from build123d import *

# Parameters (mm, degrees)
F0_W         = 119.1
F0_H         = 80
F1_DEPTH     = 5
F3_DEPTH     = 63.1
F4_W         = 6.8
F4_H         = 2
F4_W_2       = 7
F4_W_3       = 6.5
F5_DEPTH     = 4
F6_W         = 47.8
F6_H         = 2
F7_DEPTH     = 4
F8_W         = 0.5
F8_H         = 68
F9_DEPTH     = 25
F10_W        = 80
F10_H        = 5
F11_DEPTH    = 2
F12_W        = 2
F12_H        = 32.5577612221
F12_H_2      = 47.4422387779
F13_DEPTH    = 4
F14_R        = 1.99999
F15_R        = 0.5
F16_R        = 0.1
F17_T1_DEPTH = 76.00002
F17_T3_DEPTH = 1.25001
F17_T6_ANGLE = 90
F17_T8_ANGLE = 90


# Not quite as in the source:
# - a fillet or chamfer that OpenCascade refuses, or shapes differently, is made with other operations: its cross-section is extruded or revolved along the edge and cut away or added
# - a fillet or chamfer is up to 0.001 mm smaller than in the source, because OpenCascade refuses the exact size


with BuildPart() as f1:
    # F0 (on Top) → F1 (new body)
    with BuildSketch(Plane.XY):
        with Locations((59.55, 40)):
            Rectangle(F0_W, F0_H)
    extrude(amount=F1_DEPTH)

    # F2 (on face) → F3 (cut)
    with BuildSketch(Plane.XY.offset(5)):
        Polygon((64.6, 74), (64.6, 25), (64.6, 6), (65.1, 6), (65.1, 74), align=None)
    extrude(amount=-F3_DEPTH, mode=Mode.SUBTRACT)

    # F4 (on face) → F5 (join)
    with BuildSketch(Plane.XY.offset(5)):
        with Locations((32.5, 50.25)):
            Rectangle(F4_W, F4_H)
        Polygon((35.9, 49.25), (39.1217214942, 49.25), (41.1, 49.25), (41.1, 51.25), (35.9, 51.25), align=None)
        with Locations((44.6, 50.25)):
            Rectangle(F4_W_2, F4_H)
        with Locations((51.35, 50.25)):
            Rectangle(F4_W_3, F4_H)
        with Locations((19.2, 50.25)):
            Rectangle(F4_W, F4_H)
        with Locations((25.85, 50.25)):
            Rectangle(F4_W_3, F4_H)
        with Locations((58.1, 50.25)):
            Rectangle(F4_W_2, F4_H)
        with Locations((44.6, 29.75)):
            Rectangle(F4_W_2, F4_H)
        with Locations((32.5, 29.75)):
            Rectangle(F4_W, F4_H)
        with Locations((58.1, 29.75)):
            Rectangle(F4_W_2, F4_H)
        Polygon((41.1, 30.75), (39.1217214942, 30.75), (35.9, 30.75), (35.9, 28.75), (39.8, 28.75), (41.1, 28.75), align=None)
        with Locations((51.35, 29.75)):
            Rectangle(F4_W_3, F4_H)
        with Locations((25.85, 29.75)):
            Rectangle(F4_W_3, F4_H)
        with Locations((19.2, 29.75)):
            Rectangle(F4_W, F4_H)
    extrude(amount=F5_DEPTH)

    # F6 (on face) → F7 (join)
    with BuildSketch(Plane.XY.offset(5)):
        with Locations((92.1, 50.25)):
            Rectangle(F6_W, F6_H)
        with Locations((92.1, 29.75)):
            Rectangle(F6_W, F6_H)
    extrude(amount=F7_DEPTH)

    # F8 (on face) → F9 (cut)
    with BuildSketch(Plane.XY.offset(5)):
        with Locations((9.25, 40)):
            Rectangle(F8_W, F8_H)
    extrude(amount=-F9_DEPTH, mode=Mode.SUBTRACT)

    # F10 (on face) → F11 (join)
    with BuildSketch(Plane.YZ.offset(119.1)):
        with Locations((40, 2.5)):
            Rectangle(F10_W, F10_H)
    extrude(amount=F11_DEPTH)

    # F12 (on face) → F13 (join)
    with BuildSketch(Plane.XY.offset(5)):
        with Locations((120.1, 63.7211193889)):
            Rectangle(F12_W, F12_H)
        with Locations((120.1, 23.7211193889)):
            Rectangle(F12_W, F12_H_2)
    extrude(amount=F13_DEPTH)

    # F14 (radius 2 in the source; OpenCascade refuses exactly that, so slightly less here)
    f14_edges = [f1.edges().sort_by_distance(p)[0] for p in [
        (0, 80, 2.5),
        (0, 0, 2.5),
        (121.1, 80, 4.5),
        (121.1, 0, 4.5),
    ]]
    fillet(f14_edges, radius=F14_R)

    # F15
    f15_edges = [f1.edges().sort_by_distance(p)[0] for p in [
        (15.8, 49.25, 7),
        (15.8, 51.25, 7),
        (61.6, 49.25, 7),
        (61.6, 51.25, 7),
        (68.2, 49.25, 7),
        (68.2, 51.25, 7),
        (116, 49.25, 7),
        (116, 51.25, 7),
        (116, 28.75, 7),
        (116, 30.75, 7),
        (68.2, 28.75, 7),
        (68.2, 30.75, 7),
        (61.6, 28.75, 7),
        (61.6, 30.75, 7),
        (15.8, 28.75, 7),
        (15.8, 30.75, 7),
    ]]
    fillet(f15_edges, radius=F15_R)

    # F16
    f16_edges = [f1.edges().sort_by_distance(p)[0] for p in [
        (9.5, 6, 2.5),
        (9, 6, 2.5),
        (9.5, 74, 2.5),
        (9, 74, 2.5),
        (64.6, 74, 2.5),
        (65.1, 74, 2.5),
        (64.6, 6, 2.5),
        (65.1, 6, 2.5),
    ]]
    fillet(f16_edges, radius=F16_R)

    # F17: fillet of radius 0.5 on 1 edges, made by hand

    # F17_s2 → F17_t1 (cut)
    with BuildSketch(Plane.XZ.offset(-78.00001)):
        with BuildLine():
            ThreePointArc((120.6, 9), (120.9535533906, 8.8535533906), (121.1, 8.5))
            Line((121.1, 8.5), (121.1, 9))
            Line((121.1, 9), (120.6, 9))
        make_face()
    extrude(amount=F17_T1_DEPTH, mode=Mode.SUBTRACT)

    # F17_s4 → F17_t3 (cut)
    with BuildSketch(Plane.YZ.offset(117.85)):
        with BuildLine():
            ThreePointArc((80, 8.5), (79.8535533906, 8.8535533906), (79.5, 9))
            Line((79.5, 9), (80, 9))
            Line((80, 9), (80, 8.5))
        make_face()
        with BuildLine():
            ThreePointArc((0, 8.5), (0.1464466094, 8.8535533906), (0.5, 9))
            Line((0.5, 9), (0, 9))
            Line((0, 9), (0, 8.5))
        make_face()
    extrude(amount=F17_T3_DEPTH, mode=Mode.SUBTRACT)

    # F17_s5 → F17_t6 (revolve, cut)
    with BuildSketch(Plane.XZ.offset(-1.99999)):
        with BuildLine():
            ThreePointArc((120.6, 9), (120.9535533906, 8.8535533906), (121.1, 8.5))
            Line((121.1, 8.5), (121.1, 9))
            Line((121.1, 9), (120.6, 9))
        make_face()
    revolve(axis=Axis((119.10001, 1.99999, 9), (0, 0, -1)), revolution_arc=F17_T6_ANGLE, mode=Mode.SUBTRACT)

    # F17_s7 → F17_t8 (revolve, cut)
    with BuildSketch(Plane.XZ.offset(-78.00001)):
        with BuildLine():
            ThreePointArc((121.1, 8.5), (120.9535533906, 8.8535533906), (120.6, 9))
            Line((120.6, 9), (121.1, 9))
            Line((121.1, 9), (121.1, 8.5))
        make_face()
    revolve(axis=Axis((119.10001, 78.00001, 9), (0, 0, 1)), revolution_arc=F17_T8_ANGLE, mode=Mode.SUBTRACT)


solid = f1.part
Here's how the part is built. I have some questions about the finished solid (model axes, mm). A direction names the side the tool comes from. Round coordinates to 2 decimals unless told otherwise and drop trailing zeros. Order: outer loops, then holes, each group sorted by start corner. A loop starts at its lowest first (then second) coordinate and runs counter-clockwise, first axis right, second up. Notation, with made-up numbers: (-13.5, -17.5) -> (1.5, -17.5) arc R27 ccw to (1.5, 2.5) -> close; hole circle Ø9 at (82.25, 58.25). An arc over 180 degrees is marked (long way). Return JSON: item names as keys, results as strings.
Q1. I need wall thicknesses on line 1 along X through (y, z) = (15.5, 3); line 2 along Z through (x, y) = (62.5, 33); line 3 along Y through (x, z) = (31, 7.5). Which ranges of each line are inside material? Lowest first, please. Write a range as from..to.
Filled sheet:
{"line 1": "x = 0..9, 9.5..64.6, 65.1..121.1", "line 2": "z = 0..5", "line 3": "y = 28.75..30.75, 49.25..51.25"}
Q2. If we section it at B-B on x = 55: List the corners of the cut face in (y, z) for me.
Filled sheet:
{"outline": "(0, 0) -> (80, 0) -> (80, 5) -> (51.25, 5) -> (51.25, 9) -> (49.25, 9) -> (49.25, 5) -> (30.75, 5) -> (30.75, 9) -> (28.75, 9) -> (28.75, 5) -> (0, 5) -> close"}
Q3. If we mould it in two halves opening along X, with no side actions, what happens to faces 1 (the flat face through (121.1, 39, 4)), 2 (the flat face through (64.6, 40, 3)), 3 (the flat face through (92, 49.25, 7))? For each: released by +X, released by -X, zero draft, split by the parting line, or undercut.
Filled sheet:
{"face 1": "released by +X", "face 2": "undercut", "face 3": "zero draft"}
Q4. For pin 1 Ø0.5 at (y, z) = (30, 8) entering from -X; pin 2 Ø1.2 at (x, z) = (47, 7.5) entering from +Y; pin 3 Ø5 at (x, y) = (106, 65) entering from +Z, each with a flat end and sliding along its axis, tell me the tip position at first contact or that it passes through.
Filled sheet:
{"pin 1": "stops at x = 15.8", "pin 2": "stops at y = 51.25", "pin 3": "stops at z = 5"}
Q5. Which directions (+Z, -Z, +X, -X, +Y, -Y) give clear straight access to the entire face, cutting with the end or side of a thin tool? Please do faces 4 (the flat face through (39, 51.25, 7)), 5 (the flat face through (9.5, 40, 3)), 6 (the flat face through (38, 49.25, 7)), 7 (the flat face through (60, 39, 0)), 8 (the flat face through (38, 28.75, 7)).
Filled sheet:
{"face 4": "+Z, -X, +Y", "face 5": "+Z, -Z", "face 6": "+Z, -X", "face 7": "-Z, +X, -X, +Y, -Y", "face 8": "+Z, -X, -Y"}
Q6. If we section it at A-A on y = 25.5: List the corners of the cut face in (x, z) for me.
Filled sheet:
{"outline": "(0, 0) -> (9, 0) -> (9, 5) -> (0, 5) -> close; (9.5, 0) -> (64.6, 0) -> (64.6, 5) -> (9.5, 5) -> close; (65.1, 0) -> (121.1, 0) -> (121.1, 8.5) arc R0.5 ccw to (120.6, 9) -> (119.1, 9) -> (119.1, 5) -> (65.1, 5) -> close"}
